The model under review builds one solid part; all positions refer to its coordinate system, in mm. A direction names the side the tool comes from. Coordinates: 2 decimals unless noted, no trailing zeros. Loops run counter-clockwise (first coordinate to the right, second up) from the corner with the lowest first, then second, coordinate; pieces in that order, holes last. Notation, with made-up numbers: (31, 8) - (47, 8) arc R29 cw to (47, 44) - close; hole circle Ø7 at (-39, 26.5). An arc over 180 degrees is marked (long way). Use a Markdown table: item, result. Add a question column.
1) Clearance check with flat-ended pins moving along their axes: pin 1 (5 mm diameter, centred on y = -132, z = 5.5, fed in from +X); pin 2 (5 mm diameter, centred on x = 11.5, y = -155.5, fed in from +Z); pin 3 (6 mm diameter, centred on y = -57, z = 11, fed in from -X). State where each tip first meets the part, or that it passes through.
2) Add section C-C, the plane y = -60.5. Give the boundary of the cut face in (x, z), and give its area (3 significant figures).
3) Add section A-A, the plane z = 0. Give the boundary of the cut face in (x, y), and give its area (3 significant figures).
4) Add section B-B, the plane x = 0. Give the boundary of the cut face in (y, z).
5) For faces 1 (the flat face through (0, 0, 0)), 2 (the cylindrical face through (10.316, -23.706, -7.91)), list the 3-axis set-ups (+Z, -Z, +X, -X, +Y, -Y) from which the entire face can be reached by the end or side of a thin tool; tool diameter is ignored.
6) To check wall thickness, follow L1, parallel to Z at x = 0.25, y = -149; L2, parallel to X at y = -101, z = 10.5; L3, parallel to Z at x = 0, y = -92.5. State the ranges of each line that lie inside material, in increasing order. Write a range as [from, to].
7) The part is to be moulded in two halves that separate along Z. For faces 3 (the flat face through (0, -200, 0)), 4 (the cylindrical face through (-14.985, -159.44, 0.66)), say which applies: pulls with the +Z half, pulls with the -Z half, needs draft (parallel to the pull), parting line crosses it, or undercut.
```python
from build123d import *

# Parameters (mm, degrees)
F0_R     = 15
F1_DEPTH = 150
F2_R     = 15
F2_R_2   = 13
F3_DEPTH = 45
F6_R     = 15
F7_DEPTH = 50


with BuildPart() as f1:
    # F0 (on Front) → F1 (new body)
    with BuildSketch(Plane.XZ):
        Circle(F0_R)
    extrude(amount=F1_DEPTH)

    # F2 (on face) → F3 (cut)
    with BuildSketch(Plane(origin=(0, 0, 0), x_dir=(-1, 0, 0), z_dir=(0, 1, 0))):
        Circle(F2_R)
        Circle(F2_R_2, mode=Mode.SUBTRACT)
    extrude(amount=-F3_DEPTH, mode=Mode.SUBTRACT)

    # F4 (on Top) → F5 (revolve, cut)
    with BuildSketch(Plane.XY):
        Polygon((15, -45), (13, -45), (15, -120), align=None)
        Polygon((13, 0), (10, 0), (13, -3), align=None)
    revolve(axis=Axis((0, 0, 0), (0, 1, 0)), mode=Mode.SUBTRACT)

    # F6 (on face) → F7 (join)
    with BuildSketch(Plane.XZ.offset(150)):
        Circle(F6_R)
    extrude(amount=F7_DEPTH)


solid = f1.part
```
From the geometry:
| question | item | result |
|---|---|---|
| 1 | pin 1 | stops at x = 14.7 |
| 1 | pin 2 | stops at z = 12 |
| 1 | pin 3 | stops at x = -10.65 |
| 2 | outline | circle Ø26.83 at (0, 0) |
| 2 | area | 565 mm^2 |
| 3 | outline | (-15, -200) - (15, -200) - (15, -120) - (13, -45) - (13, -3) - (10, 0) - (-10, 0) - (-13, -3) - (-13, -45) - (-15, -120) - close |
| 3 | area | 5,660 mm^2 |
| 4 | outline | (-200, -15) - (-120, -15) - (-45, -13) - (-3, -13) - (0, -10) - (0, 10) - (-3, 13) - (-45, 13) - (-120, 15) - (-200, 15) - close |
| 5 | face 1 | +Z, -Z, +X, -X, +Y |
| 5 | face 2 | +Y |
| 6 | L1 | z = [-15, 15] |
| 6 | L2 | x = [-9.99, 9.99] |
| 6 | L3 | z = [-14.27, 14.27] |
| 7 | face 3 | needs draft |
| 7 | face 4 | parting line crosses it |
